Part print with two shaded views. Sizes in mm from the minimum x, y, z corner. A direction names the side the tool comes from. Coordinates: 2 decimals unless noted, no trailing zeros. Write each loop counter-clockwise with the first axis right and the second up, starting at its lowest first coordinate (ties: lowest second). Pieces come first, ordered by that corner, then holes. Notation, with made-up numbers: (-24, 0) - (9, 0) arc R20 ccw to (9, 9) - close; hole circle Ø10 at (89.25, 64.5). An arc over 180 degrees is marked (long way). Answer in a Markdown table with one row per item. Add a question column.
Q1. Band-saw the part on B-B (y = 15.25). State how many separate pieces and enclosed holes the cut face has, and give its area (3 significant figures).
Q2. 3-axis set-ups, long thin cutter, end or side, ignore diameter. For the marked faces 1 and 2: which of +Z, -Z, +X, -X, +Y, -Y reach the whole face in a straight line?
Q3. Pin check, flat tips, straight feed: pin 1 (10 mm diameter, centred on x = 19.5, y = 16.5, fed in from -Z); pin 2 (1 mm diameter, centred on y = 2.5, z = 2, fed in from -X). Stop position of each tip, or through.
Q4. Band-saw the part on C-C (y = 6.75). List the corners of the cut face in (x, z) (1 decimal), and give its area (3 significant figures).
Q5. Drill centre lines: line 1 along Y through (x, z) = (3, 0.75); line 2 along Y through (x, z) = (7.5, 1.5); line 3 along X through (y, z) = (7, 1.65) (1 decimal). Where is each one in solid material? Low to high. Write a range as from..to.
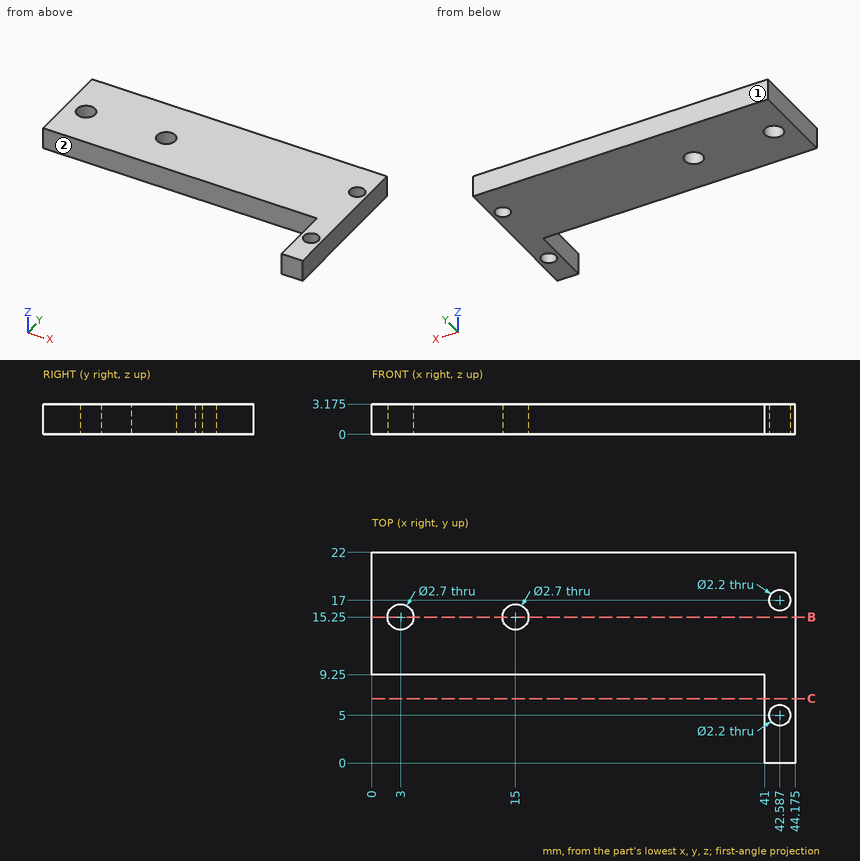
Checked values:
| question | item | result |
|---|---|---|
| 1 | separate pieces | 3 |
| 1 | enclosed holes | 0 |
| 1 | area | 123 mm² |
| 2 | face 1 | +Z, -Z, +X, -X, +Y |
| 2 | face 2 | +Z, -Z, -X, -Y |
| 3 | pin 1 | stops at z = 0 |
| 3 | pin 2 | stops at x = 41 |
| 4 | outline | (41, 0) - (44.2, 0) - (44.2, 3.2) - (41, 3.2) - close |
| 4 | area | 10.1 mm² |
| 5 | line 1 | y = 9.25..13.9, 16.6..22 |
| 5 | line 2 | y = 9.25..22 |
| 5 | line 3 | x = 41..44.2 |
